from build123d import *

# Parameters (mm, degrees)
F0_W        = 33.6334481835
F0_H        = 19.636919722
F1_DEPTH    = 25.4
F2_T1_DEPTH = 155.2122388964
F3_R        = 4.1932918126
F4_DEPTH    = 41.402
F5_DEPTH    = 6.35


# Not quite as in the source:
# - a fillet or chamfer that OpenCascade refuses, or shapes differently, is made with other operations: its cross-section is extruded or revolved along the edge and cut away or added


with BuildPart() as f1:
    # F0 (on Top) → F1 (new body)
    with BuildSketch(Plane.XY):
        with Locations((-16.8167240918, 9.818459861)):
            Rectangle(F0_W, F0_H)
    extrude(amount=F1_DEPTH)

    # F2: fillet of radius 26.9812507731 on 1 edges, made by hand

    # F2_s2 → F2_t1 (cut)
    with BuildSketch(Plane.XY.offset(-64.9061194482)):
        with BuildLine():
            ThreePointArc((-25.9624477793, 0), (-9.6862587992, 5.4621066087), (0, 19.636919722))
            Line((0, 19.636919722), (0, 0))
            Line((0, 0), (-25.9624477793, 0))
        make_face()
    extrude(amount=F2_T1_DEPTH, mode=Mode.SUBTRACT)

    # F3 (on face) → F4 (cut)
    with BuildSketch(Plane(origin=(0, 19.636919722, 0), x_dir=(-1, 0, 0), z_dir=(0, 1, 0))):
        with Locations((14.5834481835, 12.7)):
            Circle(F3_R)
    extrude(amount=-F4_DEPTH, mode=Mode.SUBTRACT)

    # F5 (add): a face of the model
    f5_faces = [f1.faces().sort_by_distance(p)[0] for p in [
        (-29.7979479814, 0, 12.7),
    ]]
    extrude(f5_faces, amount=F5_DEPTH)


solid = f1.part
Model file for the job. Use its own axes, mm. A direction names the side the tool comes from. Give positions to 0.01 mm unless a question says otherwise; leave off trailing zeros. Loops run counter-clockwise (first coordinate to the right, second up) from the corner with the lowest first, then second, coordinate; pieces in that order, holes last. Notation, with made-up numbers: (-19.75, 73) -> (-5.75, 73) arc R34 ccw to (-5.75, 110) -> close; hole circle Ø4 at (82.5, -11). An arc over 180 degrees is marked (long way). Use a Markdown table: item, result. Add a question column.
(1) Drop flat-ended pins along their axis: pin 1 Ø1.9 at (y, z) = (-2, 14) entering from +X; pin 2 Ø1 at (x, y) = (-19.5, 12) entering from -Z; pin 3 Ø4 at (x, z) = (-7, 22.5) entering from -Y; pin 4 Ø6.5 at (x, z) = (-14.58, 12.7) entering from +Y. Give the stop position or say it passes through.
(2) Mould opens along X. For faces 1 (the flat face through (-21, 19.637, 13)), 2 (the flat face through (-33.633, 7, 13)), 3 (the cylindrical face through (-18.583, 10.436, 13.96)) say: +X half, -X half, draft (parallel to the pull), parting line (faces both ways), or undercut.
(3) Slice it at B-B on x = -12. List the corners of the cut face in (y, z), and give its area (3 significant figures).
(4) Wall check: line 1 along X through (y, z) = (7.75, 12.7); line 2 along Z through (x, y) = (-13, 5.25); line 3 along X through (y, z) = (-4.5, 9.25). Give the ranges that are in metal, low to high.
(5) Slice it at C-C on z = 6.5. List the corners of the cut face in (x, y).
(6) Slice it at D-D on y = 6. List the corners of the cut face in (x, z), and give its area (3 significant figures).
(7) Tool access for faces 4 (the flat face through (-25.962, -3, 13)), 5 (the flat face through (-21, 10, 25.4)): list every direction of +Z, -Z, +X, -X, +Y, -Y with a clear straight run to the whole face (end or side of a thin tool).
(8) Slice it at A-A on z = 12.7. List the corners of the cut face in (x, y), and give its area (3 significant figures).
Filled sheet:
| question | item | result |
|---|---|---|
| 1 | pin 1 | x = -25.96 |
| 1 | pin 2 | z = 0 |
| 1 | pin 3 | y = 6 |
| 1 | pin 4 | through |
| 2 | face 1 | draft |
| 2 | face 2 | -X half |
| 2 | face 3 | undercut |
| 3 | outline | (3.89, 0) -> (19.64, 0) -> (19.64, 9.4) -> (3.89, 9.4) -> close; (3.89, 16) -> (19.64, 16) -> (19.64, 25.4) -> (3.89, 25.4) -> close |
| 3 | area | 296 mm2 |
| 4 | line 1 | -33.63 to -18.78, -10.39 to -7.04 |
| 4 | line 2 | 0 to 8.82, 16.58 to 25.4 |
| 4 | line 3 | -33.63 to -25.96 |
| 5 | outline | (-33.63, -6.35) -> (-25.96, -6.35) -> (-25.96, 0) arc R26.98 ccw to (0, 19.64) -> (-33.63, 19.64) -> close |
| 6 | outline | (-33.63, 0) -> (-9, 0) -> (-9, 25.4) -> (-33.63, 25.4) -> close; hole circle Ø8.39 at (-14.58, 12.7) |
| 6 | area | 570 mm2 |
| 7 | face 4 | +Z, -Z, +X, -Y |
| 7 | face 5 | +Z, +X, -X, +Y, -Y |
| 8 | outline | (-33.63, -6.35) -> (-25.96, -6.35) -> (-25.96, 0) arc R26.98 ccw to (-18.78, 0.97) -> (-18.78, 19.64) -> (-33.63, 19.64) -> close; (-10.39, 4.95) arc R26.98 ccw to (0, 19.64) -> (-10.39, 19.64) -> close |
| 8 | area | 433 mm2 |
